Can you work these out from the model? Positions are in its coordinate system, mm. Face numbers are marked on the shaded views. A direction names the side the tool comes from. Round coordinates to 2 decimals unless told otherwise and drop trailing zeros. Loops run counter-clockwise (first coordinate to the right, second up) from the corner with the lowest first, then second, coordinate; pieces in that order, holes last. Notation, with made-up numbers: M -18,34 L 29,34 A35 cw 29,72 Z; hole C 37,-22.5 d7. An arc over 180 degrees is marked long. Answer as CSV lines item,"result".
from build123d import *

# Parameters (mm, degrees)
F0_W     = 58.805938
F0_H     = 40.52332
F1_DEPTH = 3
F2_W     = 46.881379
F2_H     = 40.52332
F3_DEPTH = 3
F4_W     = 32.996017
F4_H     = 40.52332
F5_DEPTH = 3
F6_W     = 32.996017
F6_H     = 40.52332
F7_DEPTH = 30


with BuildPart() as f1:
    # F0 (on Top) → F1 (new body)
    with BuildSketch(Plane.XY):
        Rectangle(F0_W, F0_H)
    extrude(amount=F1_DEPTH)

    # F2 (on face) → F3 (join)
    with BuildSketch(Plane.XY.offset(3)):
        with Locations((5.962279, 0)):
            Rectangle(F2_W, F2_H)
    extrude(amount=F3_DEPTH)

    # F4 (on face) → F5 (join)
    with BuildSketch(Plane.XY.offset(6)):
        with Locations((12.90496, 0)):
            Rectangle(F4_W, F4_H)
    extrude(amount=F5_DEPTH)

    # F6 (on face) → F7 (join)
    with BuildSketch(Plane.XY.offset(9)):
        with Locations((12.90496, 0)):
            Rectangle(F6_W, F6_H)
    extrude(amount=F7_DEPTH)


solid = f1.part
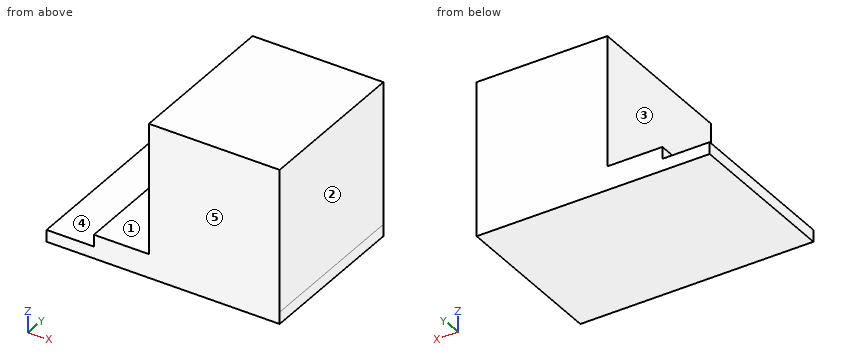
Item 1: On a 3-axis mill with a long thin cutter (end or side, diameter ignored), from which of +Z, -Z, +X, -X, +Y, -Y can I reach the whole of each face in a straight line? I mean the marked faces 4 and 5. Say none if no direction works.
Output:
face 4,"+Z, -X, +Y, -Y"
face 5,"+Z, -Z, +X, -X, -Y"
Item 2: If I drill on line 1 along X through (y, z) = (18, 9); line 2 along Z through (x, y) = (-18, -9.5); line 3 along Z through (x, y) = (-15.5, 4), over which ranges is the centre line in solid material (lowest first)? Write a range as from..to.
Output:
line 1,"x = -3.59..29.4"
line 2,"z = 0..3"
line 3,"z = 0..6"
Item 3: If we section it at A-A on y = -17.5: Write out the boundary of the cut face in (x, z).
Output:
outline,"M -29.4,0 L 29.4,0 L 29.4,39 L -3.59,39 L -3.59,6 L -17.48,6 L -17.48,3 L -29.4,3 Z"
Item 4: If we section it at C-C on z = 10: Write out the boundary of the cut face in (x, y), then the cut area to 3 significant figures.
Output:
outline,"M -3.59,-20.26 L 29.4,-20.26 L 29.4,20.26 L -3.59,20.26 Z"
area,"1,340 mm2"
Item 5: Will these pins go through, and if not, where does the flat tip stop? pin 1 (5 mm diameter, centred on y = 11, z = 29, fed in from -X); pin 2 (3 mm diameter, centred on x = -12.5, y = 13.5, fed in from +Z).
Output:
pin 1,"stops at x = -3.59"
pin 2,"stops at z = 6"
Item 6: We'd pull the mould along X, two halves only. Please class the marked faces 1, 2 and 3: released by +X, released by -X, zero draft, split by the parting line, or undercut.
Output:
face 1,"zero draft"
face 2,"released by +X"
face 3,"released by -X"
Item 7: If we section it at B-B on x = -12: Write out the boundary of the cut face in (y, z).
Output:
outline,"M -20.26,0 L 20.26,0 L 20.26,6 L -20.26,6 Z"
